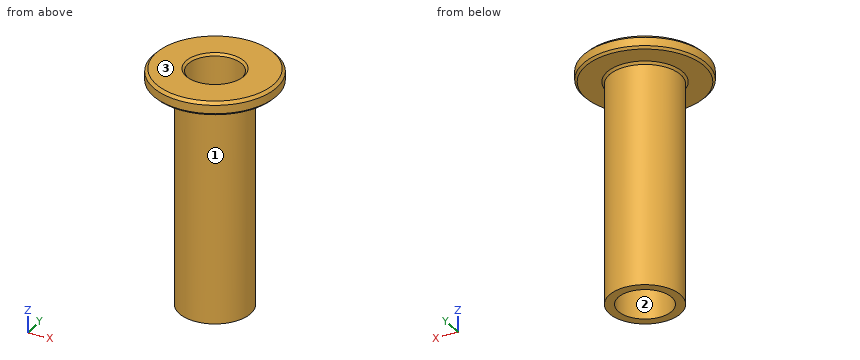
Autodesk Inventor part; units mm, degrees
ref_plane "YZ Plane" through (0, 0, 0) normal (1, 0, 0) x (0, 1, 0)
ref_plane "XZ Plane" through (0, 0, 0) normal (0, 1, 0) x (-1, 0, 0)
ref_plane "XY Plane" through (0, 0, 0) normal (0, 0, 1) x (1, 0, 0)
sketch "Esquisse1" plane through (0, 0, 0) normal (1, 0, 0) x (0, 1, 0)
  line L0 (13.35, -3) -> (8.5, -3)
  line L1 (8.5, -3) -> (8, -3.5)
  line L2 (8, -3.5) -> (8, -53)
  line L3 (8, -53) -> (6, -53)
  line L4 (6, -53) -> (6, -0.5)
  line L5 (6, -0.5) -> (6.5, 0)
  line L6 (6.5, 0) -> (13.225, 0)
  line L7 (13.225, 0) -> (13.85, -0.625)
  line L8 (13.85, -0.625) -> (13.85, -2.5)
  line L9 (13.85, -2.5) -> (13.35, -3)
  line L10 (0, 8.9692) -> (0, -52.1325)
  point P0 (0, 0)
  dimension "d0" = 3
  dimension "d3" = 0.5
  dimension "d4" = 0.5
  dimension "d5" = 0.5
  dimension "d6" = 0.5
  dimension "d7" = 0.625
  dimension "d8" = 0.625
  dimension "d9" = 0.5
  dimension "d10" = 0.5
  dimension "d12" = 50
  dimension "d15" = 12
  dimension "d16" = 27.7
  dimension "d17" = 16
revolve "Révolution1" add sketch "Esquisse1" angle 360 about axis through (0, 0, 8.9692) along (0, 0, -1)
equation "\"d4\" = d3"
equation "\"d6\" = d5"
equation "\"d8\" = d7"
equation "\"d10\" = d9"
properties part number "douille" material "Plastique ABS"
Could you check a few things on this model? Use its own coordinates, in mm. Face numbers are marked on the shaded views. Give positions to 0.01 mm unless a question says otherwise; leave off trailing zeros. Order: outer loops, then holes, each group sorted by start corner. A loop starts at its lowest first (then second) coordinate and runs counter-clockwise, first axis right, second up. Notation, with made-up numbers: (57, 0.25) -> (110, 0.25) arc R12 cw to (110, 5.25) -> close; hole circle Ø8 at (57, -9). An arc over 180 degrees is marked (long way). Return JSON: item names as keys, results as strings.
1. Imagine slicing it at C-C on z = -38.5. List the corners of the cut face in (x, y) for me, then the cut area to 3 significant figures.
Answer list:
{"outline": "circle Ø16 at (0, 0); hole circle Ø12 at (0, 0)", "area": "88.0 mm2"}
2. I need wall thicknesses on line 1 (X direction, y = 0, z = -23.5); line 2 (Z direction, x = -3, y = -11.5); line 3 (Y direction, x = 0.5, z = -48.5). Which ranges of each line are inside material? Lowest first, please. Write a range as from..to.
Answer list:
{"line 1": "x = -8..-6, 6..8", "line 2": "z = -3..0", "line 3": "y = -7.98..-5.98, 5.98..7.98"}
3. Imagine slicing it at A-A on y = 0. List the corners of the cut face in (x, z) for me (3 decimals).
Answer list:
{"outline": "(-13.85, -2.5) -> (-13.35, -3) -> (-8.5, -3) -> (-8, -3.5) -> (-8, -53) -> (-6, -53) -> (-6, -0.5) -> (-6.5, 0) -> (-13.225, 0) -> (-13.85, -0.625) -> close; (6, -53) -> (8, -53) -> (8, -3.5) -> (8.5, -3) -> (13.35, -3) -> (13.85, -2.5) -> (13.85, -0.625) -> (13.225, 0) -> (6.5, 0) -> (6, -0.5) -> close"}
4. Thinking about a two-plate mould opening in Y: for the marked faces 1, 2 and 3, which applies, pulls with the +Y half, pulls with the -Y half, needs draft (parallel to the pull), parting line crosses it, or undercut?
Answer list:
{"face 1": "parting line crosses it", "face 2": "undercut", "face 3": "needs draft"}
5. For pin 1 Ø3 at (x, y) = (10, -10) entering from -Z; pin 2 Ø3 at (x, z) = (-8, -27) entering from +Y; pin 3 Ø1.5 at (y, z) = (6, -8.5) entering from -X, each with a flat end and sliding along its axis, tell me the tip position at first contact or that it passes through.
Answer list:
{"pin 1": "stops at z = -3", "pin 2": "stops at y = 4.66", "pin 3": "stops at x = -6.04"}
